```python
from build123d import *

# Parameters (mm, degrees)
F0_R     = 69.85
F1_DEPTH = 12.7
F3_DEPTH = 3.175
F4_R     = 19.05
F5_DEPTH = 12.701


with BuildPart() as f1:
    # F0 (on Top) → F1 (new body)
    with BuildSketch(Plane.XY):
        Circle(F0_R)
    extrude(amount=-F1_DEPTH)

    # F2 (on Top) → F3 (cut)
    with BuildSketch(Plane.XY):
        Polygon((6.35, 76.042563), (-6.35, 76.042563), (-6.35, 6.35), (-75.381324, 6.35), (-75.381324, -6.35), (-6.35, -6.35), (-6.35, -74.058846), (6.35, -74.058846), (6.35, -6.35), (76.042563, -6.35), (76.042563, 6.35), (6.35, 6.35), align=None)
    extrude(amount=-F3_DEPTH, mode=Mode.SUBTRACT)

    # F4 (on Top) → F5 (cut, through all)
    with BuildSketch(Plane.XY):
        Circle(F4_R)
    extrude(amount=-F5_DEPTH, mode=Mode.SUBTRACT)


solid = f1.part
```
Verification items for the finished model (mm, model axes). A direction names the side the tool comes from. Coordinates: 2 decimals unless noted, no trailing zeros. Order: outer loops, then holes, each group sorted by start corner. A loop starts at its lowest first (then second) coordinate and runs counter-clockwise, first axis right, second up. Notation, with made-up numbers: (74, -7.75) -> (94, -7.75) arc R21 cw to (94, -1.75) -> close; hole circle Ø4 at (1, 51). An arc over 180 degrees is marked (long way). Answer as CSV lines item,"result". Start each with the question number.
1) Release check for a two-part mould opening along Y. For faces 1 (the face through (66.624, 20.981, -6.261)), 2 (the face through (43, -6.35, -2)), 3 (the face through (-31, 31, 0)) record: released by +Y, released by -Y, zero draft, split by the parting line, or undercut.
2) Cross-section at D-D, the plane y = -22.5. Record the boundary of the cut face in (x, z) (3 decimals), then the cut area to 3 significant figures.
3) Gauge pin test, flat ends, axial feed: pin 1 Ø2.5 at (x, z) = (-49, -1) entering from -Y; pin 2 Ø1 at (x, z) = (55, -1.5) entering from -Y; pin 3 Ø2 at (y, z) = (-41, -3.5) entering from +X; pin 4 Ø12 at (x, y) = (-22, 13.5) entering from +Z. Record the tip position at first contact, or that the pin passes through.
4) Set-up check for faces 4 (the face through (-44, 0, -3.175)), 5 (the face through (0, 44, -3.175)), 6 (the face through (30, -30, 0)): record each of +Z, -Z, +X, -X, +Y, -Y from which the full face is reachable in a straight line by a thin tool's end or side.
5) Material ranges on L1, parallel to X at y = 0, z = -5; L2, parallel to X at y = 46, z = -2, recorded low to high. Write a range as [from, to].
6) Cross-section at C-C, the plane z = -6.25. Record the boundary of the cut face in (x, y), then the cut area to 3 significant figures.
7) Cross-section at A-A, the plane x = 0. Record the boundary of the cut face in (y, z) (3 decimals), then the cut area to 3 significant figures.
Conclusion:
1,face 1,"split by the parting line"
1,face 2,"undercut"
1,face 3,"zero draft"
2,outline,"(-66.127, -12.7) -> (66.127, -12.7) -> (66.127, 0) -> (6.35, 0) -> (6.35, -3.175) -> (-6.35, -3.175) -> (-6.35, 0) -> (-66.127, 0) -> close"
2,area,"1,640 mm²"
3,pin 1,"stops at y = -50.98"
3,pin 2,"stops at y = -43.69"
3,pin 3,"stops at x = 57.26"
3,pin 4,"stops at z = 0"
4,face 4,"+Z, +X, -X"
4,face 5,"+Z, +Y, -Y"
4,face 6,"+Z, +X, -X, +Y, -Y"
5,L1,"x = [-69.85, -19.05], [19.05, 69.85]"
5,L2,"x = [-52.56, -6.35], [6.35, 52.56]"
6,outline,"circle Ø139.7 at (0, 0); hole circle Ø38.1 at (0, 0)"
6,area,"14,200 mm²"
7,outline,"(-69.85, -12.7) -> (-19.05, -12.7) -> (-19.05, -3.175) -> (-69.85, -3.175) -> close; (19.05, -12.7) -> (69.85, -12.7) -> (69.85, -3.175) -> (19.05, -3.175) -> close"
7,area,"968 mm²"
